```python
from build123d import *

# Parameters (mm, degrees)
CHANFREIN1_SIZE = 0.5
CHANFREIN2_SIZE = 0.3


with BuildPart() as part:
    # Esquisse1 → Révolution1 (revolve)
    with BuildSketch(Plane.XY, mode=Mode.PRIVATE) as r_volution1_sk:
        Polygon((2, 0), (2, 3.5), (6, 3.5), (6, 2.5), (4.25, 2.5), (4.25, 1.724524585), (3, 1.724524585), (3, 0), align=None)
    revolve(r_volution1_sk.sketch.rotate(Axis((0, 0, 0), (0, 1, 0)), 90), axis=Axis((0, 0, 0), (0, 1, 0)))

    # Chanfrein1
    chanfrein1_edges = [part.edges().sort_by_distance(p)[0] for p in [
        (0, 3.5, 2),
    ]]
    chamfer(chanfrein1_edges, length=CHANFREIN1_SIZE)

    # Chanfrein2
    chanfrein2_edges = [part.edges().sort_by_distance(p)[0] for p in [
        (0, 0, 3),
        (0, 1.724524585, 4.25),
    ]]
    chamfer(chanfrein2_edges, length=CHANFREIN2_SIZE)


solid = part.part
```
Design review of the part built by this model. Coordinates are the model's own, in mm. A direction names the side the tool comes from. Round coordinates to 2 decimals unless told otherwise and drop trailing zeros. Write each loop counter-clockwise with the first axis right and the second up, starting at its lowest first coordinate (ties: lowest second). Pieces come first, ordered by that corner, then holes.
Item 1: We need section D-D on z = -4.5. Write out the cut boundary in (x, y), and give its area (3 significant figures).
Item 2: Clearance check with flat-ended pins moving along their axes: pin 1 Ø1.5 at (y, z) = (1, -4.5) entering from -X; pin 2 Ø1.5 at (y, z) = (1.5, 0.5) entering from +X. State where each tip first meets the part, or that it passes through.
Item 3: We need section A-A on x = 0. Write out the cut boundary in (y, z), and give its area (3 significant figures).
Item 4: We need section B-B on z = 0. Write out the cut boundary in (x, y), and give its area (3 significant figures).
Item 5: The part is to be moulded in two halves that separate along X. For faces 3 (the cylindrical face through (2, 2, 0)), 4 (the flat face through (4, 2.5, -3)), 5 (the cylindrical face through (-1.802, 2.993, -5.723)), say which applies: +X half, -X half, draft (parallel to the pull), parting line (faces both ways), or undercut.
Item 6: For probe 1 along X at (y, z) = (1, 0); probe 2 along Y at (x, z) = (3, 0.5); probe 3 along Y at (x, z) = (-4.5, -0.5), list the stretches that pass through material, from the lowest coordinate up.
Item 7: For faces 1 (the cylindrical face through (-4.214, 2.259, 0.553)), 2 (the flat face through (0, 3.5, 3)), list the 3-axis set-ups (+Z, -Z, +X, -X, +Y, -Y) from which the entire face can be reached by the end or side of a thin tool; tool diameter is ignored.
Item 8: We need section C-C on y = 1.45. Write out the cut boundary in (x, z).
Returned:
1. outline: (-3.97, 2.5) - (3.97, 2.5) - (3.97, 3.5) - (-3.97, 3.5) - close
1. area: 7.94 mm2
2. pin 1: passes through
2. pin 2: stops at x = 4.25
3. outline: (0, -2.7) - (0.3, -3) - (1.72, -3) - (1.72, -3.95) - (2.02, -4.25) - (2.5, -4.25) - (2.5, -6) - (3.5, -6) - (3.5, -2.5) - (3, -2) - (0, -2) - close; (0, 2) - (3, 2) - (3.5, 2.5) - (3.5, 6) - (2.5, 6) - (2.5, 4.25) - (2.02, 4.25) - (1.72, 3.95) - (1.72, 3) - (0.3, 3) - (0, 2.7) - close
3. area: 14.5 mm2
4. outline: (-6, 2.5) - (-4.25, 2.5) - (-4.25, 2.02) - (-3.95, 1.72) - (-3, 1.72) - (-3, 0.3) - (-2.7, 0) - (-2, 0) - (-2, 3) - (-2.5, 3.5) - (-6, 3.5) - close; (2, 0) - (2.7, 0) - (3, 0.3) - (3, 1.72) - (3.95, 1.72) - (4.25, 2.02) - (4.25, 2.5) - (6, 2.5) - (6, 3.5) - (2.5, 3.5) - (2, 3) - close
4. area: 14.5 mm2
5. face 3: undercut
5. face 4: draft
5. face 5: parting line
6. probe 1: x = -3 to -2, 2 to 3
6. probe 2: y = 1.72 to 3.5
6. probe 3: y = 2.5 to 3.5
7. face 1: -Y
7. face 2: +Z, -Z, +X, -X, +Y
8. outline: circle Ø6 at (0, 0); hole circle Ø4 at (0, 0)
